from build123d import *

# Parameters (mm, degrees)
F1_DEPTH = 2
F4_COUNT = 6
F4_ANGLE = 300


with BuildPart() as f1:
    # F0 (on Top) → F1 (new body)
    with BuildSketch(Plane.XY):
        Polygon((-3.2329817768, 66.8248683214), (8.0453734845, 48.9121899009), (-2.093318617, 33.8490381837), (0, 13.6142224073), (0, 0), (3.7587733038, 0), (9.3085616827, 36.5094803274), (25.0811669976, 41.8303571641), (32.9873822629, 66.3811415434), (17.0520264655, 60.2824240923), (6.7185084336, 63.7288540602), (33.2126766443, 73.987826705), (19.2160885781, 78.7753090262), (32.7906534076, 84.480561316), (18.8226215541, 85.4642242193), (8.5925143212, 93.1368023157), (9.0090529993, 78.3579275012), align=None)
    extrude(amount=F1_DEPTH)

    # F2: F1 across plane


with BuildPart() as f1_1:
    add(f1.part)
    add(f1.part.mirror(Plane.YZ))

    # F4: F1 ×6 about axis
    f4_axis = Axis((0, 0, 4.1130185127), (0, 0, 1))


with BuildPart() as f1_2:
    add(f1_1.part)
    for i in range(1, F4_COUNT):
        add(f1_1.part.rotate(f4_axis, i * F4_ANGLE / (F4_COUNT - 1)))


solid = f1_2.part
Part model, mm, in its own coordinate system. A direction names the side the tool comes from. Coordinates: 2 decimals unless noted, no trailing zeros. Use a Markdown table: item, result. Add a question column.
Item 1: Which spindle directions (+Z, -Z, +X, -X, +Y, -Y) get a long thin tool onto all of the face, cutting with end or side? Do faces 1 (the flat face through (16.51, 38.94, 0.99)), 2 (the flat face through (-86.534, 20.049, 0.986)). Say none if no direction does.
Item 2: Pull direction Y, two halves, no side cores. Call faces 3 (the flat face through (33.52, 53.5, 0.99)), 4 (the flat face through (70.4, 56.557, 0.986)), 5 (the flat face through (19.78, -68.787, 0.986)): +Y half, -Y half, draft (parallel to the pull), parting line (faces both ways), or undercut.
Item 3: Band-saw the part on A-A on z = 0.3. Give the number of separate pieces and of enclosed holes in the cut face, plus the area to 3 significant figures.
Item 4: Probe probe 1 along Y at (x, z) = (5, 1.5); probe 2 along Y at (x, z) = (17.5, 0.8); probe 3 along Y at (x, z) = (-67, 1.25). List the from-to ranges inside material, lowest first.
Geometry says:
| question | item | result |
|---|---|---|
| 1 | face 1 | +Z, -Z |
| 1 | face 2 | +Z, -Z, -X |
| 2 | face 3 | undercut |
| 2 | face 4 | +Y half |
| 2 | face 5 | undercut |
| 3 | separate pieces | 1 |
| 3 | enclosed holes | 12 |
| 3 | area | 15,100 mm² |
| 4 | probe 1 | -74.58 to -53.75, -44.39 to 44.39, 53.75 to 74.58 |
| 4 | probe 2 | -86.46 to -67.9, -60.45 to -39.27, -18.75 to -2.85, 2.85 to 18.75, 39.27 to 60.45, 67.9 to 86.46 |
| 4 | probe 3 | -58.01 to -48.95, -32.99 to -19.24, -10.29 to -3.12, 3.12 to 10.29, 19.24 to 32.99, 48.95 to 58.01 |
